The model under review builds one solid part; all positions refer to its coordinate system, in mm. Face numbers are marked on the shaded views. A direction names the side the tool comes from. Coordinates: 2 decimals unless noted, no trailing zeros. Write each loop counter-clockwise with the first axis right and the second up, starting at its lowest first coordinate (ties: lowest second). Pieces come first, ordered by that corner, then holes. Notation, with made-up numbers: M 39,71 L 92,71 A35 ccw 92,103 Z; hole C -35.75,-29 d6. An arc over 180 degrees is marked long. Answer as CSV lines item,"result". Start each with the question number.
from build123d import *

# Parameters (mm, degrees)
SKETCH1_R           = 55
BOSS_EXTRUDE1_DEPTH = 40
FILLET1_R           = 10
SKETCH2_R           = 12
CUT_EXTRUDE1_DEPTH  = 658.467258663
SKETCH3_R           = 82.5
SKETCH3_R_2         = 55
CUT_EXTRUDE2_DEPTH  = 63
CHAMFER1_SIZE       = 2


with BuildPart() as part:
    # Sketch1 → Boss-Extrude1 (new, symmetric)
    with BuildSketch(Plane.XY):
        Polygon((-445, 0), (445, 0), (470, 0), (470, 15), (465, 20), (444.063252294, 20), (444.063252294, 399.999122503), (344.063252294, 499.999122503), (-344.063252294, 499.999122503), (-444.063252294, 399.999122503), (-444.063252294, 20), (-465, 20), (-470, 15), (-470, 0), align=None)
        with Locations((-316.5, 100)):
            Circle(SKETCH1_R, mode=Mode.SUBTRACT)
        with Locations(Location((316.5, 100, 0), (0, 0, 180))):
            Circle(SKETCH1_R, mode=Mode.SUBTRACT)
        with BuildLine():
            Line((-60, 457.999122503), (60, 457.999122503))
            Line((60, 457.999122503), (60, 225))
            ThreePointArc((60, 225), (0, 165), (-60, 225))
            Line((-60, 225), (-60, 457.999122503))
        make_face(mode=Mode.SUBTRACT)
    extrude(amount=BOSS_EXTRUDE1_DEPTH, both=True)

    # Fillet1
    fillet1_edges = [part.edges().sort_by_distance(p)[0] for p in [
        (444.063252294, 20, 0),
        (-444.063252294, 20, 0),
    ]]
    fillet(fillet1_edges, radius=FILLET1_R)

    # Sketch2 → Cut-Extrude1 (cut, through all)
    with BuildSketch(Plane.XZ.offset(-457.999122503)):
        with Locations(Location((0, 0, 0), (0, 0, 270))):
            Circle(SKETCH2_R)
    extrude(amount=-CUT_EXTRUDE1_DEPTH, mode=Mode.SUBTRACT)

    # Sketch3 → Cut-Extrude2 (cut)
    # profile 1 of 2: a face of its own
    with BuildSketch(Plane.XY.offset(40)):
        with Locations((-316.5, 100)):
            Circle(SKETCH3_R)
        with Locations((-316.5, 100)):
            Circle(SKETCH3_R_2, mode=Mode.SUBTRACT)
    # profile 2 of 2: a face of its own
    with BuildSketch(Plane.XY.offset(40)):
        with Locations((316.5, 100)):
            Circle(SKETCH3_R)
        with Locations(Location((316.5, 100, 0), (0, 0, 180))):
            Circle(SKETCH3_R_2, mode=Mode.SUBTRACT)
    extrude(amount=-CUT_EXTRUDE2_DEPTH, mode=Mode.SUBTRACT)

    # Chamfer1
    chamfer1_edges = [part.edges().sort_by_distance(p)[0] for p in [
        (-399, 100, -23),
        (-399, 100, 40),
        (234, 100, -23),
        (234, 100, 40),
    ]]
    chamfer(chamfer1_edges, length=CHAMFER1_SIZE)


solid = part.part
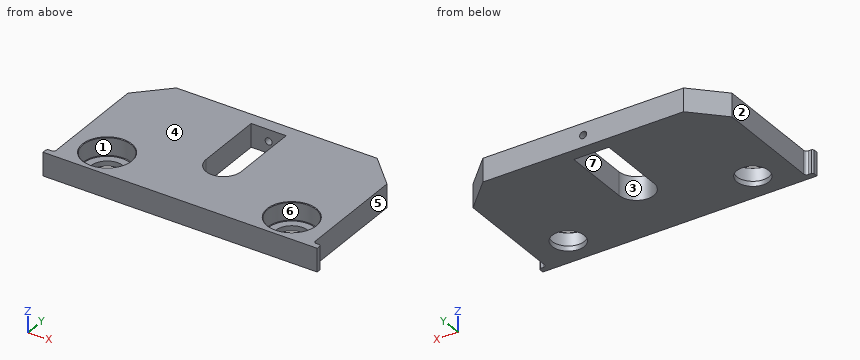
1) Take a section at C-C on z = 0. Give the boundary of the cut face in (x, y).
2) Clearance check with flat-ended pins moving along their axes: pin 1 Ø5 at (y, z) = (275.5, -9.5) entering from +X; pin 2 Ø12 at (x, z) = (458.5, -7.5) entering from +Y; pin 3 Ø1.5 at (y, z) = (244.5, 6) entering from -X. State where each tip first meets the part, or that it passes through.
3) Take a section at A-A on x = 0. Give the boundary of the cut face in (y, z).
4) Tool access review of the marked faces 5, 6 and 7: name each direction out of +Z, -Z, +X, -X, +Y, -Y from which nothing blocks a thin tool from reaching the whole face with its end or side.
5) Take a section at B-B on y = 100. Give the boundary of the cut face in (x, z), and give its area (3 significant figures).
6) Take a section at D-D on y = 297. Give the boundary of the cut face in (x, z).
7) To check wall thickness, follow line 1 (X direction, y = 388.5, z = -22); line 2 (Y direction, x = -316, z = 21); line 3 (X direction, y = 145.5, z = -3). State the ranges of each line that lie inside material, in increasing order. Write a range as [from, to].
8) Mouldability with a two-part tool opening along X and no side actions: class the marked faces 1, 2, 3 and 4 as +X half, -X half, draft (parallel to the pull), parting line (faces both ways), or undercut.
Results:
1,outline,"M -470,0 L 470,0 L 470,15 L 465,20 L 454.06,20 A10 cw 444.06,30 L 444.06,400 L 344.06,500 L 12,500 L 12,458 L 60,458 L 60,225 A60 cw -60,225 L -60,458 L -12,458 L -12,500 L -344.06,500 L -444.06,400 L -444.06,30 A10 cw -454.06,20 L -465,20 L -470,15 Z; hole C -316.5,100 d165; hole C 316.5,100 d165"
2,pin 1,"stops at x = 444.06"
2,pin 2,"stops at y = 20.12"
2,pin 3,"stops at x = -444.06"
3,outline,"M 0,-40 L 165,-40 L 165,40 L 0,40 Z; M 458,-40 L 500,-40 L 500,-12 L 458,-12 Z; M 458,12 L 500,12 L 500,40 L 458,40 Z"
4,face 5,"+Z, -Z, +X, +Y"
4,face 6,"+Z"
4,face 7,"+Z, -Z"
5,outline,"M -444.06,-40 L -371.5,-40 L -371.5,-23 L -397,-23 L -399,-21 L -399,38 L -401,40 L -444.06,40 Z; M -261.5,-40 L 261.5,-40 L 261.5,-23 L 236,-23 L 234,-21 L 234,38 L 232,40 L -232,40 L -234,38 L -234,-21 L -236,-23 L -261.5,-23 Z; M 371.5,-40 L 444.06,-40 L 444.06,40 L 401,40 L 399,38 L 399,-21 L 397,-23 L 371.5,-23 Z"
5,area,"46,500 mm²"
6,outline,"M -444.06,-40 L -60,-40 L -60,40 L -444.06,40 Z; M 60,-40 L 444.06,-40 L 444.06,40 L 60,40 Z"
7,line 1,"x = [-444.06, -60], [60, 444.06]"
7,line 2,"y = [0, 17.5], [182.5, 500]"
7,line 3,"x = [-444.06, -385.32], [-247.68, 247.68], [385.32, 444.06]"
8,face 1,"undercut"
8,face 2,"-X half"
8,face 3,"undercut"
8,face 4,"draft"
